The drawing under review shows one solid part. Ordinate dimensions are in mm from its lowest x, y, z. A direction names the side the tool comes from. Give positions to 0.01 mm unless a question says otherwise; leave off trailing zeros. Write each loop counter-clockwise with the first axis right and the second up, starting at its lowest first coordinate (ties: lowest second). Pieces come first, ordered by that corner, then holes. Notation, with made-up numbers: M 66.25,-37 L 81.25,-37 A19 cw 81.25,-9 Z; hole C 52.5,-26 d11. An arc over 180 degrees is marked long. One line per item, written item: value. Start each with the question number.
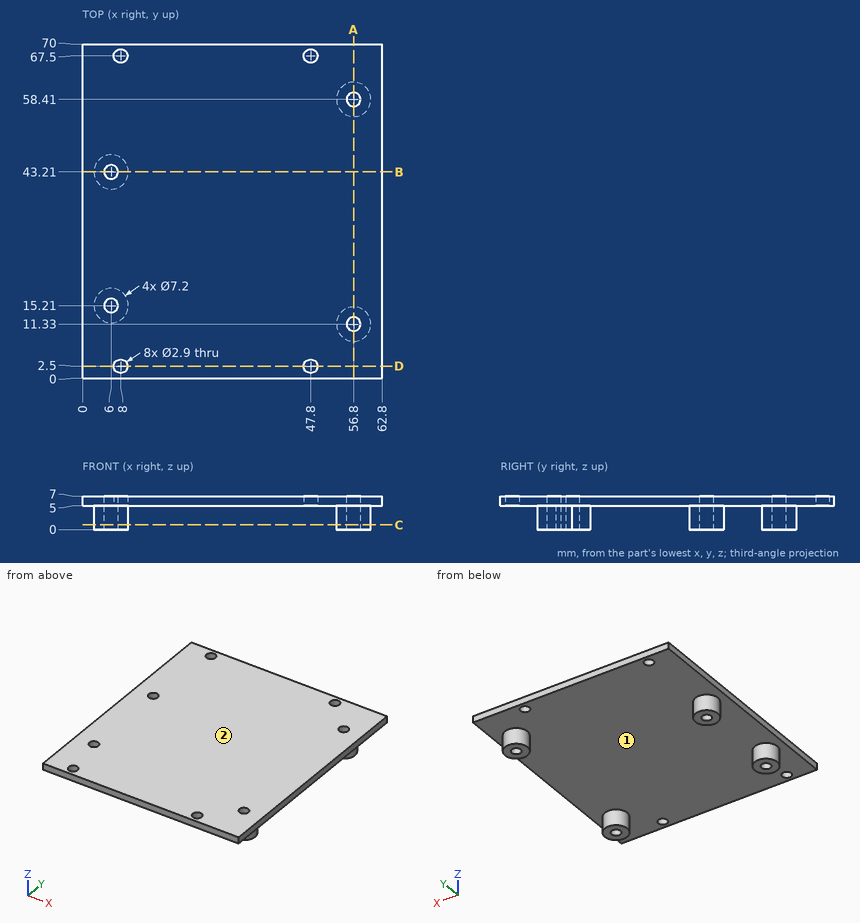
Q1. Take a section at B-B, the plane y = 43.21. Give the boundary of the cut face in (x, z), then the cut area to 3 significant figures.
Q2. Take a section at A-A, the plane x = 56.8. Give the boundary of the cut face in (y, z).
Q3. For P1, Ø4, axis at x = 8, y = 2.5, coming from the -Z side; P2, Ø2, axis at x = 8.5, z = 3, coming from the -Y side; P3, Ø1.7, axis at x = 47.8, y = 2.5, coming from the +Z side, all flat-tipped, find the tip position at first contact; note any pin that passes through.
Q4. Take a section at D-D, the plane y = 2.5. Give the boundary of the cut face in (x, z).
Q5. Take a section at C-C, the plane z = 1. Give the boundary of the cut face in (x, y), then the cut area to 3 significant figures.
Q6. Machinability: for the marked faces 1 and 2, which of the approach directions +Z, -Z, +X, -X, +Y, -Y give a long, thin tool a straight path to every point of the face, cutting with its end or side? Answer none if there is none.
Q7. Wall thickness on line 1 (Y direction, x = 8, z = 6.1); line 2 (X direction, y = 67.5, z = 6.05); line 3 (Y direction, x = 6, z = 5.5): over which ranges is each line inside the solid? List them lowest first. Write a range as from..to.
Results list:
1. outline: M 0,5 L 2.4,5 L 2.4,0 L 4.55,0 L 4.55,7 L 0,7 Z; M 7.45,0 L 9.6,0 L 9.6,5 L 62.8,5 L 62.8,7 L 7.45,7 Z
1. area: 141 mm^2
2. outline: M 0,5 L 7.73,5 L 7.73,0 L 9.88,0 L 9.88,7 L 0,7 Z; M 12.78,0 L 14.93,0 L 14.93,5 L 54.81,5 L 54.81,0 L 56.96,0 L 56.96,7 L 12.78,7 Z; M 59.86,0 L 62.01,0 L 62.01,5 L 70,5 L 70,7 L 59.86,7 Z
3. P1: stops at z = 5
3. P2: stops at y = 11.94
3. P3: passes through
4. outline: M 0,5 L 6.55,5 L 6.55,7 L 0,7 Z; M 9.45,5 L 46.35,5 L 46.35,7 L 9.45,7 Z; M 49.25,5 L 62.8,5 L 62.8,7 L 49.25,7 Z
5. outline: C 6,15.21 d7.2; C 6,43.21 d7.2; C 56.8,11.33 d7.2; C 56.8,58.41 d7.2; hole C 6,15.21 d2.9; hole C 6,43.21 d2.9; hole C 56.8,11.33 d2.9; hole C 56.8,58.41 d2.9
5. area: 136 mm^2
6. face 1: -Z
6. face 2: +Z, +X, -X, +Y, -Y
7. line 1: y = 0..1.05, 3.95..66.05, 68.95..70
7. line 2: x = 0..6.55, 9.45..46.35, 49.25..62.8
7. line 3: y = 0..13.76, 16.66..41.76, 44.66..70
